Geometry check sheet. Reference: drawing and pictorial views, mm from the part's lowest x, y, z. Round coordinates to 2 decimals unless told otherwise and drop trailing zeros. Loops run counter-clockwise (first coordinate to the right, second up) from the corner with the lowest first, then second, coordinate; pieces in that order, holes last. Notation, with made-up numbers: (29, -4) - (39, -4) arc R16 ccw to (39, 4) - close; hole circle Ø7 at (-37.75, 54). An arc over 180 degrees is marked (long way). Put each result on its own line as item: value. Start each with the question number.
Item 1: Material ranges on line 1 along Z through (x, y) = (105, 0.95); line 2 along Z through (x, y) = (104, 0.8) (1 decimal); line 3 along X through (y, z) = (2.65, 59) (1 decimal), recorded low to high.
Item 2: Section check A-A, the plane x = 105. Record the cut outline in (y, z).
Item 3: Gauge pin test, flat ends, axial feed: pin 1 Ø2 at (y, z) = (3, 77) entering from -X; pin 2 Ø6.5 at (x, z) = (147.85, 129.74) entering from +Y; pin 3 Ø1.5 at (y, z) = (1, 26) entering from -X (1 decimal); pin 4 Ø1.2 at (y, z) = (1.5, 75) entering from +X. Record the tip position at first contact, or that the pin passes through.
Item 4: Section check D-D, the plane z = 129.74. Record the cut outline in (x, y).
Item 5: Section check B-B, the plane y = 0.6. Record the cut outline in (x, z) (1 decimal).
Item 6: Section check C-C, the plane z = 73. Record the cut outline in (x, y) (1 decimal), and give its area (3 significant figures).
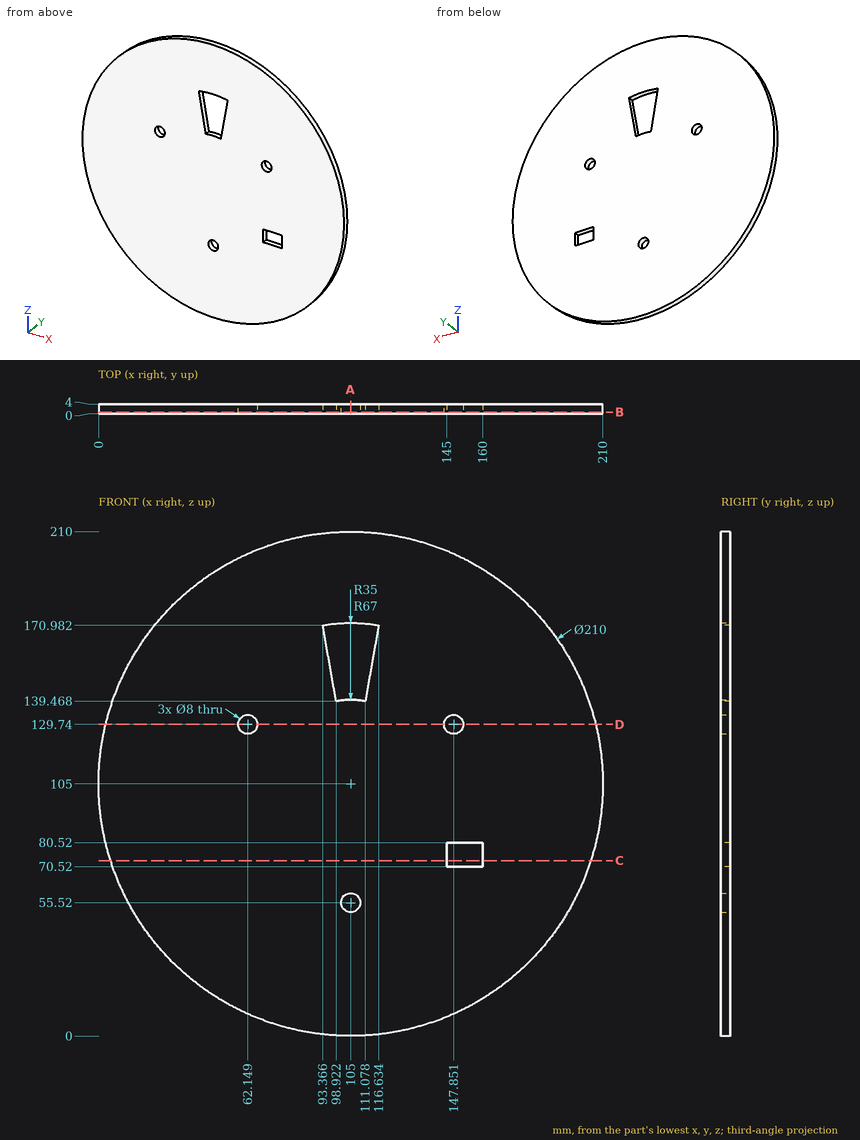
Check result:
1. line 1: 0 to 51.52, 59.52 to 140, 172 to 210
1. line 2: 0 to 51.6, 59.4 to 140, 172 to 210
1. line 3: 10.6 to 103, 107 to 199.4
2. outline: (0, 0) - (4, 0) - (4, 51.52) - (0, 51.52) - close; (0, 59.52) - (4, 59.52) - (4, 140) - (0, 140) - close; (0, 172) - (4, 172) - (4, 210) - (0, 210) - close
3. pin 1: x = 3.53
3. pin 2: through
3. pin 3: x = 35
3. pin 4: x = 205.8
4. outline: (2.96, 0) - (58.15, 0) - (58.15, 4) - (2.96, 4) - close; (66.15, 0) - (143.85, 0) - (143.85, 4) - (66.15, 4) - close; (151.85, 0) - (207.04, 0) - (207.04, 4) - (151.85, 4) - close
5. outline: circle Ø210 at (105, 105); hole circle Ø8 at (62.1, 129.7); hole (93.4, 171) - (98.9, 139.5) arc R35 cw to (111.1, 139.5) - (116.6, 171) arc R67 ccw to start; hole circle Ø8 at (105, 55.5); hole circle Ø8 at (147.9, 129.7); hole (145, 70.5) - (160, 70.5) - (160, 80.5) - (145, 80.5) - close
6. outline: (5, 0) - (145, 0) - (145, 4) - (5, 4) - close; (160, 0) - (205, 0) - (205, 4) - (160, 4) - close
6. area: 740 mm²
